Design review of the part built by this model. Coordinates are the model's own, in mm. Coordinates: 2 decimals unless noted, no trailing zeros. Write each loop counter-clockwise with the first axis right and the second up, starting at its lowest first coordinate (ties: lowest second). Pieces come first, ordered by that corner, then holes. Notation, with made-up numbers: (17.5, -26.5) - (65.5, -26.5) arc R29 ccw to (65.5, -1.5) - close; hole circle Ø9 at (-10, 52). An arc over 180 degrees is marked (long way). Answer as a JSON object with one key per item and string values.
```python
from build123d import *

# Parameters (mm, degrees)
EXTRUDE_THIN1_DEPTH                   = 137.50025
EXTRUDE_THIN1_DEPTH_BACK              = 213.5
BOSS_EXTRUDE1_DEPTH                   = 212.50025
BOSS_EXTRUDE1_DEPTH_BACK              = 288.5
SKETCH3_OUTSIDE_W                     = 604.182
SKETCH3_OUTSIDE_H                     = 156.652
SKETCH3_OUTSIDE_W_2                   = 500
SKETCH3_OUTSIDE_H_2                   = 100
CUT_EXTRUDE1_DEPTH                    = 47.972186303
F_1_4_20_TAPPED_HOLE1_D               = 5.1054
F_1_4_20_TAPPED_HOLE1_DEPTH           = 16.51
F_1_4_20_TAPPED_HOLE1_TIP             = 1.533816902
F_1_4_20_TAPPED_HOLE1_ON_FACE_2_D     = 5.1054
F_1_4_20_TAPPED_HOLE1_ON_FACE_2_DEPTH = 16.51
F_1_4_20_TAPPED_HOLE1_ON_FACE_2_TIP   = 1.533816902


with BuildPart() as part:
    # Sketch1 → Extrude-Thin1 (new body, two sides)
    with BuildSketch(Plane.XY) as extrude_thin1_sk:
        with BuildLine():
            Line((-1, 29.097280522), (-1, 77.801426037))
            ThreePointArc((-1, 77.801426037), (-1.350622843, 78.7652373), (-2.238576202, 79.27846957))
            Line((-2.238576202, 79.27846957), (-14.558703222, 81.459024393))
            ThreePointArc((-14.558703222, 81.459024393), (-15.894736772, 81.028505528), (-16.289731153, 79.68154169))
            Line((-16.289731153, 79.68154169), (-16.133756175, 78.918587006))
            ThreePointArc((-16.133756175, 78.918587006), (-16.425245764, 77.689683446), (-17.55197675, 77.119028185))
            Line((-17.55197675, 77.119028185), (-31.176844121, 76.652024665))
            ThreePointArc((-31.176844121, 76.652024665), (-32.394172227, 75.953136676), (-32.500485503, 74.55348328))
            Line((-32.500485503, 74.55348328), (-32.189291755, 73.839630008))
            ThreePointArc((-32.189291755, 73.839630008), (-32.21890818, 72.576976846), (-33.20237149, 71.784531227))
            Line((-33.20237149, 71.784531227), (-46.048094305, 68.590520727))
            ThreePointArc((-46.048094305, 68.590520727), (-47.095522717, 67.648327863), (-46.899674591, 66.2531658))
            Line((-46.899674591, 66.2531658), (-20.221033316, 29.533166286))
            ThreePointArc((-20.221033316, 29.533166286), (-19.7411642, 29.106506164), (-19.126852316, 28.919599404))
            Line((-19.126852316, 28.919599404), (-2.619344492, 27.602035762))
            ThreePointArc((-2.619344492, 27.602035762), (-1.482408908, 27.995233168), (-1, 29.097280522))
        make_face()
        with BuildLine():
            Line((-1.27, 29.097280522), (-1.27, 77.801426037))
            ThreePointArc((-1.27, 77.801426037), (-1.557510731, 78.591751273), (-2.285632486, 79.012601734))
            Line((-2.285632486, 79.012601734), (-14.605759506, 81.193156557))
            ThreePointArc((-14.605759506, 81.193156557), (-15.701307017, 80.840131088), (-16.025202409, 79.735620741))
            Line((-16.025202409, 79.735620741), (-15.869227431, 78.972666057))
            ThreePointArc((-15.869227431, 78.972666057), (-16.213185147, 77.522559856), (-17.542727709, 76.849186648))
            Line((-17.542727709, 76.849186648), (-31.16759508, 76.382183127))
            ThreePointArc((-31.16759508, 76.382183127), (-32.165804128, 75.809094976), (-32.252981014, 74.661379192))
            Line((-32.252981014, 74.661379192), (-31.941787266, 73.94752592))
            ThreePointArc((-31.941787266, 73.94752592), (-31.976734648, 72.457595189), (-33.137221353, 71.522509358))
            Line((-33.137221353, 71.522509358), (-45.982944168, 68.328498858))
            ThreePointArc((-45.982944168, 68.328498858), (-46.841835466, 67.55590071), (-46.681240003, 66.411867819))
            Line((-46.681240003, 66.411867819), (-20.002598727, 29.691868304))
            ThreePointArc((-20.002598727, 29.691868304), (-19.609106053, 29.342007004), (-19.105370308, 29.188743461))
            Line((-19.105370308, 29.188743461), (-2.597862483, 27.871179818))
            ThreePointArc((-2.597862483, 27.871179818), (-1.665575304, 28.193601692), (-1.27, 29.097280522))
        make_face(mode=Mode.SUBTRACT)
    extrude(amount=EXTRUDE_THIN1_DEPTH)
    extrude(extrude_thin1_sk.sketch, amount=-EXTRUDE_THIN1_DEPTH_BACK)


with BuildPart() as body_2:
    # Sketch2 → Boss-Extrude1 (new body, two sides)
    with BuildSketch(Plane.XY) as boss_extrude1_sk:
        with BuildLine():
            Line((-46.68124, 66.411867814), (-20.002598727, 29.691868304))
            ThreePointArc((-20.002598727, 29.691868304), (-19.609106053, 29.342007004), (-19.105370308, 29.188743461))
            Line((-19.105370308, 29.188743461), (-2.597862483, 27.871179818))
            ThreePointArc((-2.597862483, 27.871179818), (-1.665575304, 28.193601692), (-1.27, 29.097280522))
            Line((-1.27, 29.097280522), (-1.27, 77.801426032))
            Line((-1.27, 77.801426032), (-1.27, 77.950492716))
            ThreePointArc((-1.27, 77.950492716), (-1.551343626, 78.723865476), (-2.263847169, 79.135688695))
            Line((-2.263847169, 79.135688695), (-14.583974189, 81.316243518))
            ThreePointArc((-14.583974189, 81.316243518), (-15.79085783, 80.927341477), (-16.14766942, 79.710584143))
            Line((-16.14766942, 79.710584143), (-15.991694442, 78.947629459))
            ThreePointArc((-15.991694442, 78.947629459), (-16.311361359, 77.599931889), (-17.547009673, 76.974113285))
            Line((-17.547009673, 76.974113285), (-31.171877043, 76.507109765))
            ThreePointArc((-31.171877043, 76.507109765), (-32.271530099, 75.875780948), (-32.367566426, 74.611427381))
            Line((-32.367566426, 74.611427381), (-32.056372677, 73.897574109))
            ThreePointArc((-32.056372677, 73.897574109), (-32.088852024, 72.512864474), (-33.167383454, 71.643815779))
            Line((-33.167383454, 71.643815779), (-46.013106268, 68.449805279))
            ThreePointArc((-46.013106268, 68.449805279), (-46.895812164, 67.655785195), (-46.730763849, 66.480031545))
            Line((-46.730763849, 66.480031545), (-46.68124, 66.411867814))
        make_face()
    extrude(amount=BOSS_EXTRUDE1_DEPTH)
    extrude(boss_extrude1_sk.sketch, amount=-BOSS_EXTRUDE1_DEPTH_BACK)

    # Sketch3 outside → Cut-Extrude1 (cut, through all)
    with BuildSketch(Plane(origin=(0, 0, 0), x_dir=(0, 0, -1), z_dir=(1, 0, 0))):
        with Locations((38, 54.602)):
            Rectangle(SKETCH3_OUTSIDE_W, SKETCH3_OUTSIDE_H)
        with Locations((37.999875, 53.523886616)):
            Rectangle(SKETCH3_OUTSIDE_W_2, SKETCH3_OUTSIDE_H_2, mode=Mode.SUBTRACT)
    extrude(amount=-CUT_EXTRUDE1_DEPTH, mode=Mode.SUBTRACT)

    # 1/4-20 Tapped Hole1
    with Locations(Plane(origin=(-13.27, 66.023886616, 212.000125), x_dir=(1, 0, 0), z_dir=(0, 0, 1))):
        with Locations((0, 0), (0, -25)):
            Hole(F_1_4_20_TAPPED_HOLE1_D / 2, depth=F_1_4_20_TAPPED_HOLE1_DEPTH)
            with Locations((0, 0, -(F_1_4_20_TAPPED_HOLE1_DEPTH + F_1_4_20_TAPPED_HOLE1_TIP / 2))):  # 118° drill point
                Cone(0, F_1_4_20_TAPPED_HOLE1_D / 2, F_1_4_20_TAPPED_HOLE1_TIP, mode=Mode.SUBTRACT)

    # 1/4-20 Tapped Hole1 on face 2
    with Locations(Plane(origin=(-13.27, 66.023886616, -287.999875), x_dir=(-1, 0, 0), z_dir=(0, 0, -1))):
        with Locations((0, 0), (0, -25)):
            Hole(F_1_4_20_TAPPED_HOLE1_ON_FACE_2_D / 2, depth=F_1_4_20_TAPPED_HOLE1_ON_FACE_2_DEPTH)
            with Locations((0, 0, -(F_1_4_20_TAPPED_HOLE1_ON_FACE_2_DEPTH + F_1_4_20_TAPPED_HOLE1_ON_FACE_2_TIP / 2))):  # 118° drill point
                Cone(0, F_1_4_20_TAPPED_HOLE1_ON_FACE_2_D / 2, F_1_4_20_TAPPED_HOLE1_ON_FACE_2_TIP, mode=Mode.SUBTRACT)


solid = body_2.part
```
(1) Take a section at A-A, the plane z = -80. Write out the cut boundary in (x, y) (1 decimal), and give its area (3 significant figures).
Solved:
{"outline": "(-46.7, 66.5) - (-20, 29.7) arc R1.2 ccw to (-19.1, 29.2) - (-2.6, 27.9) arc R1.2 ccw to (-1.3, 29.1) - (-1.3, 78) arc R1.2 ccw to (-2.3, 79.1) - (-14.6, 81.3) arc R1.4 ccw to (-16.1, 79.7) - (-16, 78.9) arc R1.6 cw to (-17.5, 77) - (-31.2, 76.5) arc R1.4 ccw to (-32.4, 74.6) - (-32.1, 73.9) arc R1.6 cw to (-33.2, 71.6) - (-46, 68.4) arc R1.3 ccw to start", "area": "1,620 mm^2"}
(2) For pin 1 (3 mm diameter, centred on x = -13.27, y = 66.02, fed in from -Z); pin 2 (4.5 mm diameter, centred on x = -13.27, y = 41.02, fed in from +Z); pin 3 (8 mm diameter, centred on y = 41.5, z = 25, fed in from -X), all flat-tipped, find the tip position at first contact; note any pin that passes through.
Solved:
{"pin 1": "stops at z = -270.86", "pin 2": "stops at z = 195.31", "pin 3": "stops at x = -31.49"}
(3) To check wall thickness, follow line 1 (Y direction, x = -13.27, z = 206.75); line 2 (Y direction, x = -13, z = -279); line 3 (X direction, y = 45, z = 118.5). State the ranges of each line that lie inside material, in increasing order. Write a range as from..to.
Solved:
{"line 1": "y = 28.72..38.47, 43.58..63.47, 68.58..81.08", "line 2": "y = 28.7..38.49, 43.56..63.49, 68.56..81.04", "line 3": "x = -31.12..-1.27"}
